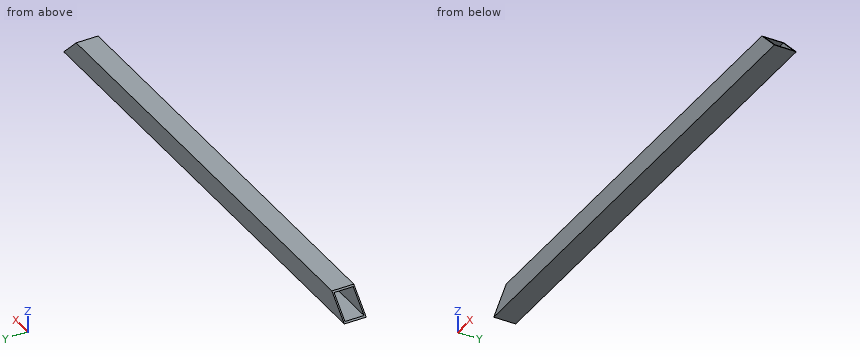
from build123d import *

# Parameters (mm, degrees)
SKETCH1_W               = 19.05
SKETCH1_H               = 19.05
BOSS_EXTRUDE1_DEPTH     = 215
SKETCH2_W               = 16.65
SKETCH2_H               = 16.65
CUT_EXTRUDE1_DEPTH      = 431.210938087
CUT_EXTRUDE2_DEPTH      = 216.421566353
CUT_EXTRUDE2_DEPTH_BACK = 216.421566353


with BuildPart() as part:
    # Sketch1 → Boss-Extrude1 (new, symmetric)
    with BuildSketch(Plane(origin=(0, 0, 0), x_dir=(0, 0, -1), z_dir=(1, 0, 0))):
        Rectangle(SKETCH1_W, SKETCH1_H)
    extrude(amount=BOSS_EXTRUDE1_DEPTH, both=True)

    # Sketch2 → Cut-Extrude1 (cut, through all)
    with BuildSketch(Plane.ZY.offset(215)):
        Rectangle(SKETCH2_W, SKETCH2_H)
    extrude(amount=-CUT_EXTRUDE1_DEPTH, mode=Mode.SUBTRACT)

    # Sketch3 → Cut-Extrude2 (cut, two sides: drawn at the far end of the back side and taken through both)
    with BuildSketch(Plane(origin=(0, 0, 0), x_dir=(1, 0, 0), z_dir=(0, 1, 0)).offset(-CUT_EXTRUDE2_DEPTH_BACK)):
        Polygon((-215, 9.525), (-215, -9.525), (-195.95, -9.525), align=None)
        Polygon((215, -9.525), (195.95, -9.525), (215, 9.525), align=None)
    extrude(amount=CUT_EXTRUDE2_DEPTH + CUT_EXTRUDE2_DEPTH_BACK, mode=Mode.SUBTRACT)


solid = part.part
Source: CAD feature listing. Evaluate the final solid. Frame: model axes, mm. Round coordinates to 2 decimals unless told otherwise and drop trailing zeros. Loops run counter-clockwise (first coordinate to the right, second up) from the corner with the lowest first, then second, coordinate; pieces in that order, holes last. Notation, with made-up numbers: (-26, -18) -> (31, -18) arc R22 cw to (31, 9) -> close; hole circle Ø6 at (27, 6). An arc over 180 degrees is marked (long way). Answer as a JSON object with one key per item and string values. Group by question number.
Q1. Section query C-C (z = 3). Output: boundary loops of the cut face in (x, y) (3 decimals).
Q2. Section query B-B (x = -179). Output: boundary loops of the cut face in (y, z) (3 decimals), plus the area to 3 significant figures.
Q3. Section query A-A (y = -4). Output: boundary loops of the cut face in (x, z) (3 decimals), plus the area to 3 significant figures.
Q4. Ray query, line 1 (Y direction, x = -136, z = 1) (3 decimals); line 2 (X direction, y = -5.75, z = -8.5) (3 decimals). Return the intervals inside material, ascending. Write a range as from..to.
Completed:
{
 "1": {"outline": "(-202.475, -9.525) -> (202.475, -9.525) -> (202.475, -8.325) -> (-202.475, -8.325) -> close; (-202.475, 8.325) -> (202.475, 8.325) -> (202.475, 9.525) -> (-202.475, 9.525) -> close"},
 "2": {"outline": "(-9.525, -9.525) -> (9.525, -9.525) -> (9.525, 9.525) -> (-9.525, 9.525) -> close; hole (-8.325, -8.325) -> (8.325, -8.325) -> (8.325, 8.325) -> (-8.325, 8.325) -> close", "area": "85.7 mm²"},
 "3": {"outline": "(-215, -9.525) -> (215, -9.525) -> (213.8, -8.325) -> (-213.8, -8.325) -> close; (-197.15, 8.325) -> (197.15, 8.325) -> (195.95, 9.525) -> (-195.95, 9.525) -> close", "area": "986 mm²"},
 "4": {"line 1": "-9.525..-8.325, 8.325..9.525", "line 2": "-213.975..213.975"}
}
